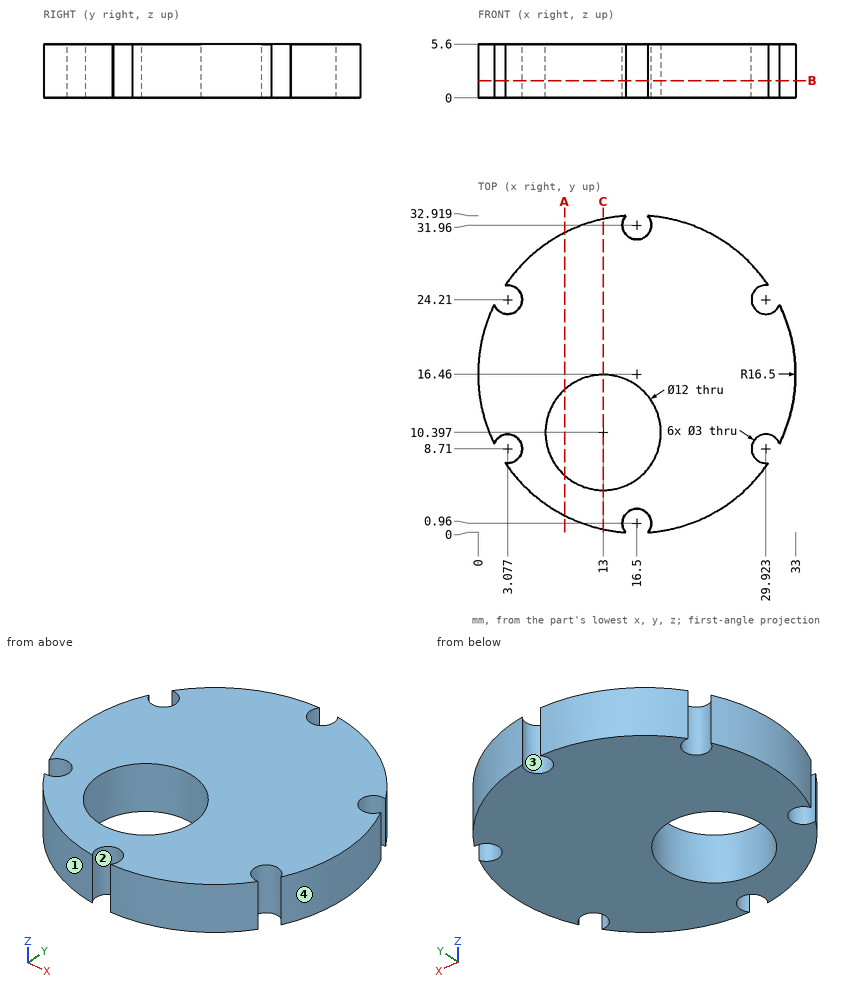
Here's the drawing with two shaded views (mm, measured from the low corner). I have some questions. Round coordinates to 2 decimals unless told otherwise and drop trailing zeros. Loops run counter-clockwise (first coordinate to the right, second up) from the corner with the lowest first, then second, coordinate; pieces in that order, holes last. Notation, with made-up numbers: (57, 83) - (91, 83) arc R21 ccw to (91, 98) - close; hole circle Ø3 at (10.5, 83). An arc over 180 degrees is marked (long way). Use CSV: the item, a comma, the result in double quotes. Start each with the question number.
1) If we section it at A-A on x = 9: Write out the boundary of the cut face in (y, z) (1 decimal).
2) For pin 1 Ø3 at (y, z) = (7, 2.5) entering from -X; pin 2 Ø5 at (x, y) = (29.92, 8.71) entering from -Z; pin 3 Ø1.5 at (y, z) = (13, 2) entering from +X; pin 4 Ø1.5 at (x, z) = (19.5, 1) entering from -Y, each with a flat end and sliding along its axis, tell me the tip position at first contact or that it passes through.
3) If we section it at C-C on x = 13: Write out the boundary of the cut face in (y, z) (1 decimal).
4) If we section it at B-B on z = 1.8: Write out the boundary of the cut face in (x, y).
5) Please list where these lines run through material, in increasing order: probe 1 along Y at (x, z) = (4, 2.2) (1 decimal); probe 2 along X at (y, z) = (23.5, 4.55) (1 decimal); probe 3 along X at (y, z) = (7, 4.35) (1 decimal). Write a range as [from, to].
6) We'd pull the mould along X, two halves only. Please class the marked faces 1, 2, 3 and 4: released by +X, released by -X, zero draft, split by the parting line, or undercut.
Geometry results:
1,outline,"(1.8, 0) - (5.9, 0) - (5.9, 5.6) - (1.8, 5.6) - close; (14.9, 0) - (31.2, 0) - (31.2, 5.6) - (14.9, 5.6) - close"
2,pin 1,"stops at x = 2.82"
2,pin 2,"stops at z = 0"
2,pin 3,"stops at x = 32.78"
2,pin 4,"stops at y = 0.11"
3,outline,"(0.3, 0) - (4.4, 0) - (4.4, 5.6) - (0.3, 5.6) - close; (16.4, 0) - (32.6, 0) - (32.6, 5.6) - (16.4, 5.6) - close"
4,outline,"(1.67, 9.23) arc R1.5 cw (long way) to (2.82, 7.23) arc R16.5 ccw to (15.35, 0) arc R1.5 cw (long way) to (17.65, 0) arc R16.5 ccw to (30.18, 7.23) arc R1.5 cw (long way) to (31.33, 9.23) arc R16.5 ccw to (31.33, 23.69) arc R1.5 cw (long way) to (30.18, 25.69) arc R16.5 ccw to (17.65, 32.92) arc R1.5 cw (long way) to (15.35, 32.92) arc R16.5 ccw to (2.82, 25.69) arc R1.5 cw (long way) to (1.67, 23.69) arc R16.5 ccw to start; hole circle Ø12 at (13, 10.4)"
5,probe 1,"y = [5.7, 7.5], [9.9, 23], [25.4, 27.2]"
5,probe 2,"x = [1.6, 1.8], [4.4, 28.6], [31.2, 31.4]"
5,probe 3,"x = [3, 8.1], [17.9, 30]"
6,face 1,"released by -X"
6,face 2,"undercut"
6,face 3,"undercut"
6,face 4,"released by +X"
